CAD build for the part. Positions are in the model's coordinates, mm. Face numbers are marked on the shaded views. Give positions to 0.01 mm unless a question says otherwise; leave off trailing zeros. Order: outer loops, then holes, each group sorted by start corner. A loop starts at its lowest first (then second) coordinate and runs counter-clockwise, first axis right, second up.
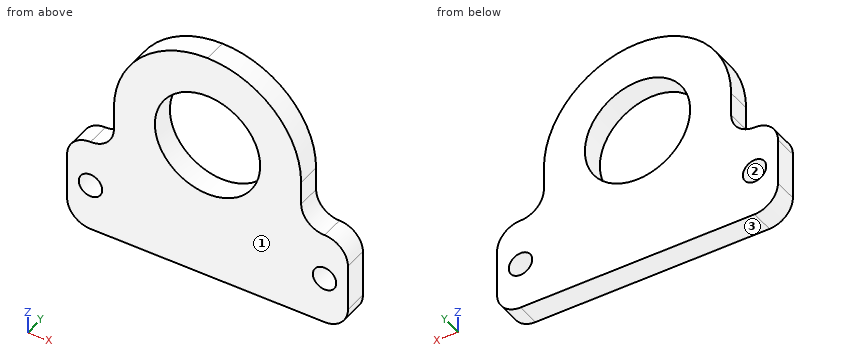
from build123d import *

# Parameters (mm, degrees)
F0_R     = 3.175
F0_R_2   = 14.2875
F1_DEPTH = 6.35


with BuildPart() as f1:
    # F0 (on Front) → F1 (new body)
    with BuildSketch(Plane.XZ):
        with BuildLine():
            Line((-6.35, -63.5), (0, -63.5))
            Line((0, -63.5), (50.8, -63.5))
            Line((50.8, -63.5), (57.15, -63.5))
            ThreePointArc((57.15, -63.5), (61.640128, -61.640128), (63.5, -57.15))
            Line((63.5, -57.15), (63.5, -44.45))
            ThreePointArc((63.5, -44.45), (61.640128, -39.959872), (57.15, -38.1))
            ThreePointArc((57.15, -38.1), (52.659872, -36.240128), (50.8, -31.75))
            Line((50.8, -31.75), (50.8, -25.4))
            ThreePointArc((50.8, -25.4), (43.360512, -7.439488), (25.4, 0))
            ThreePointArc((25.4, 0), (7.439488, -7.439488), (0, -25.4))
            Line((0, -25.4), (0, -31.75))
            ThreePointArc((0, -31.75), (-1.859872, -36.240128), (-6.35, -38.1))
            ThreePointArc((-6.35, -38.1), (-10.840128, -39.959872), (-12.7, -44.45))
            Line((-12.7, -44.45), (-12.7, -57.15))
            ThreePointArc((-12.7, -57.15), (-10.840128, -61.640128), (-6.35, -63.5))
        make_face()
        with Locations((-6.35, -50.8)):
            Circle(F0_R, mode=Mode.SUBTRACT)
        with Locations((57.15, -50.8)):
            Circle(F0_R, mode=Mode.SUBTRACT)
        with Locations((25.4, -25.4)):
            Circle(F0_R_2, mode=Mode.SUBTRACT)
    extrude(amount=F1_DEPTH)


solid = f1.part
1. Saw through at B-B on z = -12.5. Give the cut face in (x, y).
2. Pin check, flat tips, straight feed: P1, Ø1, axis at x = 21.5, y = -3, coming from the +Z side; P2, Ø3, axis at y = -4, z = -27, coming from the +X side; P3, Ø5.5, axis at x = 57.15, z = -50.8, coming from the +Y side; P4, Ø1.9, axis at y = -3.5, z = -29.5, coming from the -X side. Stop position of each tip, or through.
3. Saw through at A-A on y = -1.25. State how many separate pieces and enclosed holes the cut face has, plus the area to 3 significant figures.
4. Wall check: line 1 (Z direction, x = 25.4, y = -4.5); line 2 (Z direction, x = 57, y = -4); line 3 (X direction, y = -0.5, z = -29). Give the ranges that are in metal, low to high.
5. Saw through at D-D on x = 7. Give the cut face in (y, z).
6. Saw through at C-C on x = 58.5. Give the cut face in (y, z).
7. Mould opens along Z. For the marked faces 1, 2 and 3 say: released by +Z, released by -Z, zero draft, split by the parting line, or undercut.
Reported:
1. outline: (3.52, -6.35) - (19.26, -6.35) - (19.26, 0) - (3.52, 0) - close; (31.54, -6.35) - (47.28, -6.35) - (47.28, 0) - (31.54, 0) - close
2. P1: stops at z = -0.23
2. P2: stops at x = 50.8
2. P3: passes through
2. P4: stops at x = 0
3. separate pieces: 1
3. enclosed holes: 3
3. area: 2,870 mm2
4. line 1: z = -63.5 to -39.69, -11.11 to 0
4. line 2: z = -63.5 to -53.97, -47.63 to -38.1
4. line 3: x = 0 to 11.57, 39.23 to 50.8
5. outline: (-6.35, -63.5) - (0, -63.5) - (0, -7.89) - (-6.35, -7.89) - close
6. outline: (-6.35, -63.35) - (0, -63.35) - (0, -53.67) - (-6.35, -53.67) - close; (-6.35, -47.93) - (0, -47.93) - (0, -38.25) - (-6.35, -38.25) - close
7. face 1: zero draft
7. face 2: undercut
7. face 3: released by -Z
